from build123d import *

# Parameters (mm, degrees)
BOSS_EXTRUDE1_DEPTH = 6.35
SKETCH2_R           = 5
CUT_EXTRUDE1_DEPTH  = 6.35
SKETCH3_R           = 11
CUT_EXTRUDE2_DEPTH  = 7.3500001
SKETCH4_W           = 15
SKETCH4_H           = 110
BOSS_EXTRUDE3_DEPTH = 6.35


with BuildPart() as part:
    # Sketch1 → Boss-Extrude1 (new body)
    with BuildSketch(Plane(origin=(0, 0, 0), x_dir=(1, 0, 0), z_dir=(0, 1, 0))):
        with BuildLine():
            Line((0, 110), (0, 0))
            add(Edge.make_bspline(
                [(0, 0), (67.941176471, 0), (105, 25)],
                knots=[1.570796327, 1.570796327, 1.570796327, 2.564661308, 2.564661308, 2.564661308], degree=2, weights=[1, 0.879049073, 1]))
            Line((105, 25), (105, 85))
            add(Edge.make_bspline(
                [(105, 85), (67.941176471, 110), (0, 110)],
                knots=[3.718523999, 3.718523999, 3.718523999, 4.71238898, 4.71238898, 4.71238898], degree=2, weights=[1, 0.879049073, 1]))
        make_face()
    extrude(amount=BOSS_EXTRUDE1_DEPTH)

    # Sketch2 → Cut-Extrude1 (cut)
    with BuildSketch(Plane(origin=(0, 0, 0), x_dir=(1, 0, 0), z_dir=(0, 1, 0))):
        with Locations((95, 67.5)):
            Circle(SKETCH2_R)
        with Locations((95, 42.5)):
            Circle(SKETCH2_R)
    extrude(amount=CUT_EXTRUDE1_DEPTH, mode=Mode.SUBTRACT)

    # Sketch3 → Cut-Extrude2 (cut, through all)
    with BuildSketch(Plane(origin=(0, 0, 0), x_dir=(1, 0, 0), z_dir=(0, 1, 0))):
        with Locations((65, 55)):
            Circle(SKETCH3_R)
    extrude(amount=CUT_EXTRUDE2_DEPTH, mode=Mode.SUBTRACT)

    # Sketch4 → Boss-Extrude3 (add)
    with BuildSketch(Plane(origin=(0, 0, 0), x_dir=(1, 0, 0), z_dir=(0, 1, 0))):
        with Locations((-7.5, 55)):
            Rectangle(SKETCH4_W, SKETCH4_H)
    extrude(amount=BOSS_EXTRUDE3_DEPTH)


solid = part.part
The listing builds one solid part. Answer for the finished solid, in the listing's coordinates (mm). Round coordinates to 2 decimals unless told otherwise and drop trailing zeros. Write each loop counter-clockwise with the first axis right and the second up, starting at its lowest first coordinate (ties: lowest second). Pieces come first, ordered by that corner, then holes. Notation, with made-up numbers: (3.5, -0.75) - (53.5, -0.75) arc R19 cw to (53.5, 14.25) - close; hole circle Ø9 at (-37, 39). An arc over 180 degrees is marked (long way). Use one line per item in the form item = value. Start each with the question number.
Item 1: Flat-ended cylindrical pins translate along their axes: pin 1 Ø9 at (x, z) = (95, -67.5) entering from +Y; pin 2 Ø2 at (x, y) = (50.5, 1) entering from +Z; pin 3 Ø2 at (x, y) = (36.5, 2) entering from +Z; pin 4 Ø1.5 at (x, y) = (44, 3.5) entering from -Z. Find the tip coordinate at first contact, or state that the pin passes through.
Item 2: Determine the mould class of faces 1 (the cylindrical face through (97.688, 3.131, -46.716)), 2 (the flat face through (-8, 3, -110)), 3 (the flat face through (105, 3, -55)), 4 (the flat face through (-8, 3, 0)) for opening direction Z: +Z half, -Z half, draft (parallel to the pull), parting line (faces both ways), or undercut.
Item 3: A cutting plane is placed at A-A (z = -67.5). Write down the section's boundary in (x, y), plus the area to 4 significant figures.
Item 4: A cutting plane is placed at C-C (y = 2). Give the number of separate pieces and of enclosed holes in the cut face, plus the area to 3 significant figures.
Item 5: Find the intervals of material crossed by line 1 (X direction, y = 2.5, z = -67.5); line 2 (Z direction, x = 95, y = 4); line 3 (X direction, y = 1.5, z = -55), in increasing order. Write a range as [from, to].
Item 6: A cutting plane is placed at B-B (z = -55). Write down the section's boundary in (x, y).
The answers:
q1.pin_1 = through
q1.pin_2 = -4.48
q1.pin_3 = -2.25
q1.pin_4 = -106.62
q2.face_1 = undercut
q2.face_2 = -Z half
q2.face_3 = draft
q2.face_4 = +Z half
q3.outline = (-15, 0) - (90, 0) - (90, 6.35) - (-15, 6.35) - close; (100, 0) - (105, 0) - (105, 6.35) - (100, 6.35) - close
q3.area = 698.5 mm^2
q4.separate_pieces = 1
q4.enclosed_holes = 3
q4.area = 11,100 mm^2
q5.line_1 = [-15, 90], [100, 105]
q5.line_2 = [-90.85, -72.5], [-62.5, -47.5], [-37.5, -19.15]
q5.line_3 = [-15, 54], [76, 105]
q6.outline = (-15, 0) - (54, 0) - (54, 6.35) - (-15, 6.35) - close; (76, 0) - (105, 0) - (105, 6.35) - (76, 6.35) - close
